Geometry check sheet. Reference: drawing and pictorial views, mm from the part's lowest x, y, z. Round coordinates to 2 decimals unless told otherwise and drop trailing zeros. Loops run counter-clockwise (first coordinate to the right, second up) from the corner with the lowest first, then second, coordinate; pieces in that order, holes last. Notation, with made-up numbers: (-16, 4.25) - (36, 4.25) arc R32 ccw to (36, 31.25) - close; hole circle Ø2 at (26.5, 62). An arc over 180 degrees is marked (long way). Return JSON: item names as keys, results as strings.
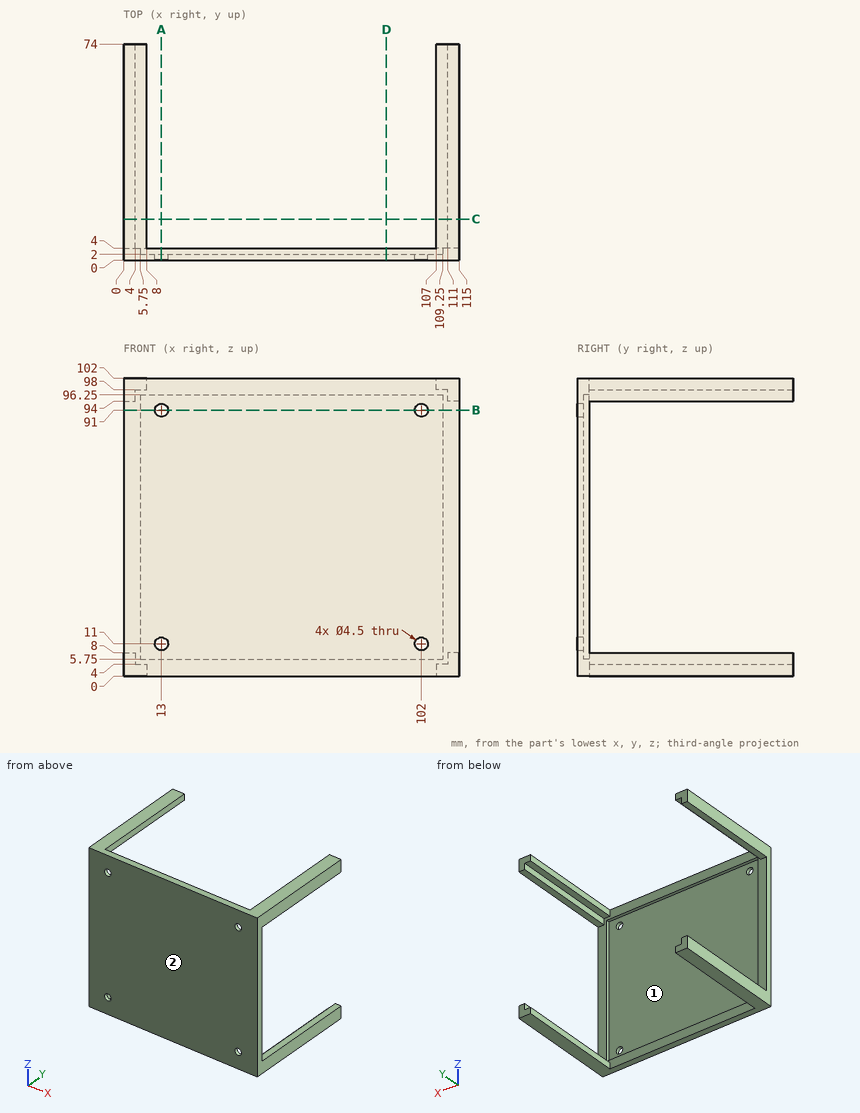
Q1. Depth check by flat-ended pin: P1, Ø4.5, axis at y = 32, z = 96, coming from the -X side; P2, Ø6, axis at x = 13.5, y = 19, coming from the -Z side; P3, Ø6, axis at x = 20, z = 45, coming from the +Y side. Enter the tip coordinate at first touch or a pass-through.
Answer key:
{"P1": "stops at x = 0", "P2": "passes through", "P3": "stops at y = 2"}
Q2. Draft check along Z on the marked faces 1 and 2. Enter one of: released by +Z, released by -Z, zero draft, split by the parting line, or undercut.
Answer key:
{"face 1": "undercut", "face 2": "zero draft"}
Q3. Sectioned sample at C-C (y = 14). Enter the section's corners in (x, z), plus the area to 3 significant figures.
Answer key:
{"outline": "(0, 0) - (8, 0) - (8, 4) - (4, 4) - (4, 8) - (0, 8) - close; (0, 94) - (4, 94) - (4, 98) - (8, 98) - (8, 102) - (0, 102) - close; (107, 0) - (115, 0) - (115, 8) - (111, 8) - (111, 4) - (107, 4) - close; (107, 98) - (111, 98) - (111, 94) - (115, 94) - (115, 102) - (107, 102) - close", "area": "192 mm²"}
Q4. Sectioned sample at A-A (x = 13). Enter the section's corners in (y, z).
Answer key:
{"outline": "(0, 0) - (4, 0) - (4, 5.75) - (2, 5.75) - (2, 8.75) - (0, 8.75) - close; (0, 13.25) - (2, 13.25) - (2, 88.75) - (0, 88.75) - close; (0, 93.25) - (2, 93.25) - (2, 96.25) - (4, 96.25) - (4, 102) - (0, 102) - close"}
Q5. Sectioned sample at B-B (z = 91). Enter the section's corners in (x, y).
Answer key:
{"outline": "(0, 0) - (10.75, 0) - (10.75, 2) - (5.75, 2) - (5.75, 4) - (0, 4) - close; (15.25, 0) - (99.75, 0) - (99.75, 2) - (15.25, 2) - close; (104.25, 0) - (115, 0) - (115, 4) - (109.25, 4) - (109.25, 2) - (104.25, 2) - close"}
Q6. Sectioned sample at D-D (x = 90). Enter the section's corners in (y, z).
Answer key:
{"outline": "(0, 0) - (4, 0) - (4, 5.75) - (2, 5.75) - (2, 96.25) - (4, 96.25) - (4, 102) - (0, 102) - close"}
Q7. Scan lines: probe 1 along X at (y, z) = (1, 91); probe 2 along Y at (x, z) = (62, 68.5); probe 3 along Y at (x, z) = (28, 97.5). Record each from-to range of solid material in increasing order. Write a range as [from, to].
Answer key:
{"probe 1": "x = [0, 10.75], [15.25, 99.75], [104.25, 115]", "probe 2": "y = [0, 2]", "probe 3": "y = [0, 4]"}
